Here's how the part is built. I have some questions about the finished solid (model axes, mm). Coordinates: 2 decimals unless noted, no trailing zeros. Order: outer loops, then holes, each group sorted by start corner. A loop starts at its lowest first (then second) coordinate and runs counter-clockwise, first axis right, second up. Notation, with made-up numbers: (85.25, -11.5) - (139.25, -11.5) arc R9 ccw to (139.25, -6.5) - close; hole circle Ø10 at (52.25, 17). An arc over 180 degrees is marked (long way). Answer as CSV lines item,"result". Start each with the question number.
Item 1: Imagine slicing it at D-D on y = -4.5. List the corners of the cut face in (x, z) for me, and give its area (3 significant figures).
Item 2: Imagine slicing it at A-A on y = -1.25. List the corners of the cut face in (x, z) for me.
Item 3: I'm going to push flat-ended pins straight in: pin 1 (2 mm diameter, centred on x = 2.5, z = 6, fed in from -Y); pin 2 (5 mm diameter, centred on x = 0, z = 5, fed in from -Y). Where does each tip first touch, or does it pass through?
Item 4: We'd pull the mould along Z, two halves only. Please class faces 1 (the face through (0, -2, 10)), 2 (the face through (-15, -1, 5)), 3 (the face through (0, -1, 7)): pulls with the +Z half, pulls with the -Z half, needs draft (parallel to the pull), parting line crosses it, or undercut.
Item 5: I need wall thicknesses on line 1 (Z direction, x = 0, y = 0.75); line 2 (Y direction, x = 11.6, z = 6); line 3 (X direction, y = -2, z = 5). Which ranges of each line are inside material? Lowest first, please.
Item 6: Imagine slicing it at C-C on x = -11.6. List the corners of the cut face in (y, z) for me, and give its area (3 significant figures).
Item 7: Imagine slicing it at B-B on z = 5. List the corners of the cut face in (x, y) for me.
from build123d import *

# Parameters (mm, degrees)
SKETCH1_R                     = 1.5
BOSS_EXTRUDE1_DEPTH           = 10
CSK_FOR_M4_SFHCS1_D           = 4
CSK_FOR_M4_SFHCS1_DEPTH       = 19
CSK_FOR_M4_SFHCS1_CSINK_D     = 7.9
CSK_FOR_M4_SFHCS1_CSINK_ANGLE = 90
CSK_FOR_M4_SFHCS1_TIP         = 1.201721238


with BuildPart() as part:
    # Sketch1 → Boss-Extrude1 (new body)
    with BuildSketch(Plane.XY):
        Polygon((-15, 2.5), (-15, -5), (-13, -7), (13, -7), (15, -5), (15, 2.5), align=None)
        with Locations((11.6, -1.25)):
            Circle(SKETCH1_R, mode=Mode.SUBTRACT)
        with Locations((-11.6, -1.25)):
            Circle(SKETCH1_R, mode=Mode.SUBTRACT)
    extrude(amount=BOSS_EXTRUDE1_DEPTH)

    # CSK for M4 SFHCS1
    with Locations(Plane(origin=(1278.247292614, -7, -931.083024415), x_dir=(1, 0, 0), z_dir=(0, -1, 0))):
        with Locations((-1278.247292614, 936.083024415)):
            CounterSinkHole(CSK_FOR_M4_SFHCS1_D / 2, CSK_FOR_M4_SFHCS1_CSINK_D / 2, depth=CSK_FOR_M4_SFHCS1_DEPTH, counter_sink_angle=CSK_FOR_M4_SFHCS1_CSINK_ANGLE)
            with Locations((0, 0, -(CSK_FOR_M4_SFHCS1_DEPTH + CSK_FOR_M4_SFHCS1_TIP / 2))):  # 118° drill point
                Cone(0, CSK_FOR_M4_SFHCS1_D / 2, CSK_FOR_M4_SFHCS1_TIP, mode=Mode.SUBTRACT)


solid = part.part
Responses:
1,outline,"(-15, 0) - (15, 0) - (15, 10) - (-15, 10) - close; hole circle Ø4 at (0, 5)"
1,area,"287 mm^2"
2,outline,"(-15, 0) - (-13.1, 0) - (-13.1, 10) - (-15, 10) - close; (-10.1, 0) - (10.1, 0) - (10.1, 10) - (-10.1, 10) - close; (13.1, 0) - (15, 0) - (15, 10) - (13.1, 10) - close; hole circle Ø4 at (0, 5)"
3,pin 1,"stops at y = -6.74"
3,pin 2,"stops at y = -5.55"
4,face 1,"pulls with the +Z half"
4,face 2,"needs draft"
4,face 3,"undercut"
5,line 1,"z = 0 to 3, 7 to 10"
5,line 2,"y = -7 to -2.75, 0.25 to 2.5"
5,line 3,"x = -15 to -12.9, -10.3 to -2, 2 to 10.3, 12.9 to 15"
6,outline,"(-7, 0) - (-2.75, 0) - (-2.75, 10) - (-7, 10) - close; (0.25, 0) - (2.5, 0) - (2.5, 10) - (0.25, 10) - close"
6,area,"65.0 mm^2"
7,outline,"(-15, -5) - (-13, -7) - (-3.95, -7) - (-2, -5.05) - (-2, 2.5) - (-15, 2.5) - close; (2, -5.05) - (3.95, -7) - (13, -7) - (15, -5) - (15, 2.5) - (2, 2.5) - close; hole circle Ø3 at (-11.6, -1.25); hole circle Ø3 at (11.6, -1.25)"
